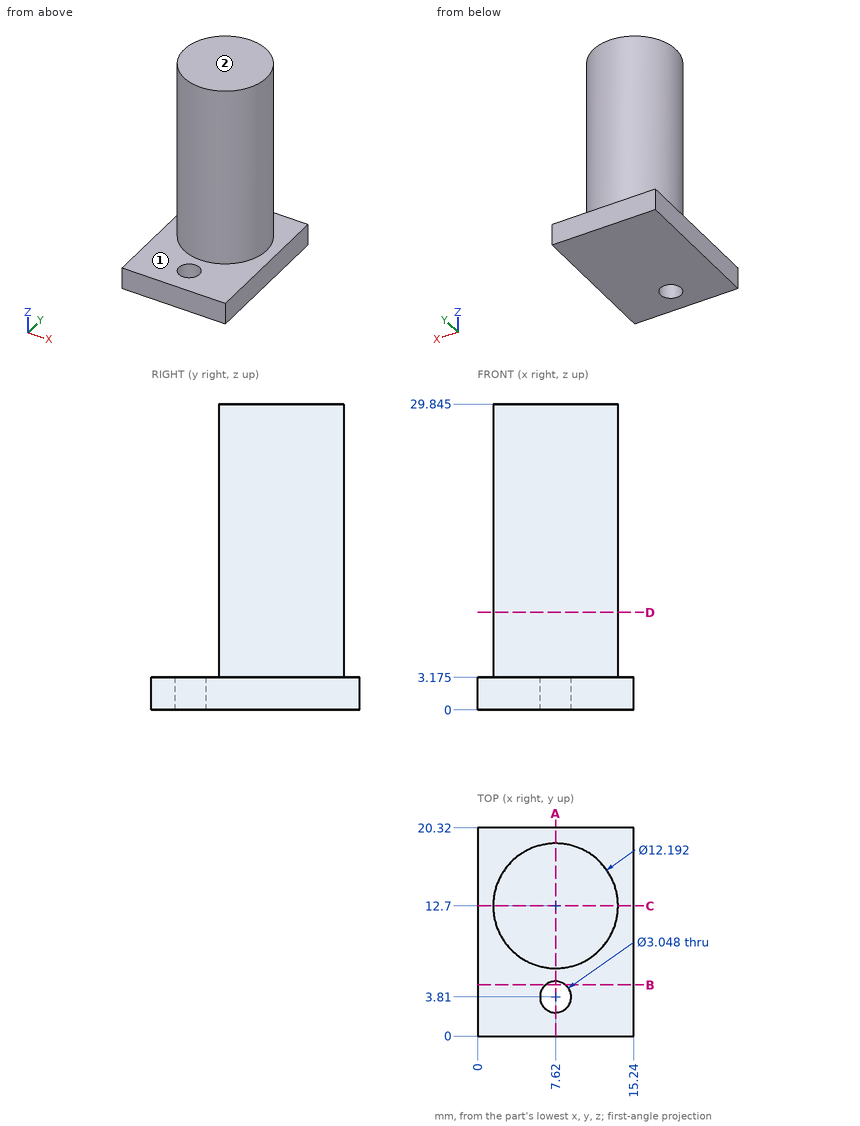
Geometry: see drawing. Coordinates: mm, zero at the bounding-box minimum. A direction names the side the tool comes from. Coordinates: 2 decimals unless noted, no trailing zeros. Loops run counter-clockwise (first coordinate to the right, second up) from the corner with the lowest first, then second, coordinate; pieces in that order, holes last. Notation, with made-up numbers: M -12.5,40 L 46.5,40 A12 cw 46.5,50 Z; hole C -34,-1 d1. An arc over 180 degrees is marked long. Put each result on its own line as item: value. Start each with the question number.
1) Cut plane C-C on y = 12.7. Return the cut outline in (x, z) (3 decimals).
2) Cut plane B-B on y = 5. Return the cut outline in (x, z) (3 decimals).
3) Cut plane A-A on x = 7.62. Return the cut outline in (y, z) (3 decimals), then the cut area to 3 significant figures.
4) Ray query, L1, parallel to Y at x = 7.62, z = 1.75; L2, parallel to Z at x = 10.75, y = 3 (3 decimals); L3, parallel to X at y = 9.75, z = 14.25. Return the intervals inside material, ascending. Write a range as from..to.
5) Cut plane D-D on z = 9.5. Return the cut outline in (x, y).
6) Reachability of the marked faces 1 and 2 from +Z, -Z, +X, -X, +Y, -Y: full face, straight path, thin tool, end or side. Return the list, or none.
7) Contact query for flat-ended pins moving along their axis: pin 1 Ø5 at (x, y) = (7.62, 3.81) entering from +Z (3 decimals); pin 2 Ø4 at (y, z) = (15, 24) entering from -X; pin 3 Ø1.5 at (y, z) = (12, 17) entering from +X. Output: stop coordinate, or through.
The answers:
1. outline: M 0,0 L 15.24,0 L 15.24,3.175 L 13.716,3.175 L 13.716,29.845 L 1.524,29.845 L 1.524,3.175 L 0,3.175 Z
2. outline: M 0,0 L 6.668,0 L 6.668,3.175 L 0,3.175 Z; M 8.572,0 L 15.24,0 L 15.24,3.175 L 8.572,3.175 Z
3. outline: M 0,0 L 2.286,0 L 2.286,3.175 L 0,3.175 Z; M 5.334,0 L 20.32,0 L 20.32,3.175 L 18.796,3.175 L 18.796,29.845 L 6.604,29.845 L 6.604,3.175 L 5.334,3.175 Z
3. area: 380 mm²
4. L1: y = 0..2.29, 5.33..20.32
4. L2: z = 0..3.175
4. L3: x = 2.29..12.95
5. outline: C 7.62,12.7 d12.19
6. face 1: +Z
6. face 2: +Z, +X, -X, +Y, -Y
7. pin 1: stops at z = 3.175
7. pin 2: stops at x = 1.53
7. pin 3: stops at x = 13.72
